Geometry: final body of the model. Coordinates: model frame, mm. Face numbers are marked on the shaded views. Round coordinates to 2 decimals unless told otherwise and drop trailing zeros. Loops run counter-clockwise (first coordinate to the right, second up) from the corner with the lowest first, then second, coordinate; pieces in that order, holes last. Notation, with made-up numbers: (12, 89.25) - (53, 89.25) arc R15 ccw to (53, 97.25) - close; hole circle Ø9 at (80, 9.5). An arc over 180 degrees is marked (long way). Answer as CSV lines item,"result".
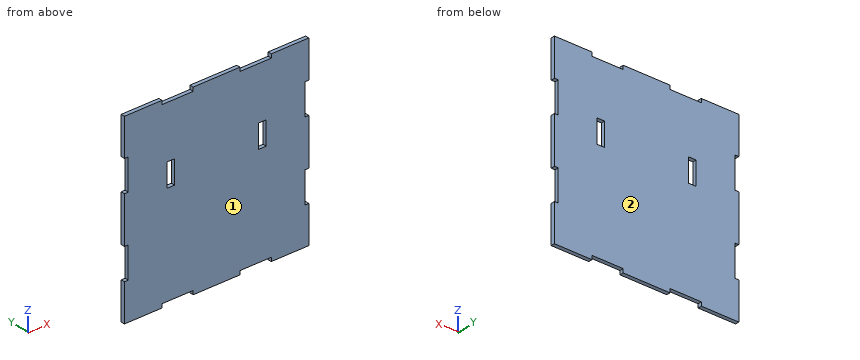
from build123d import *

# Parameters (mm, degrees)
CROQUIS1_W              = 4.84
CROQUIS1_H              = 15
SALIENTE_EXTRUIR1_DEPTH = 2.44


with BuildPart() as part:
    # Croquis1 → Saliente-Extruir1 (new body)
    with BuildSketch(Plane(origin=(0, 0, 0), x_dir=(1, 0, 0), z_dir=(0, 1, 0))):
        Polygon((-59, -59), (-35, -59), (-35, -56.56), (-15, -56.56), (-15, -59), (15, -59), (15, -56.56), (35, -56.56), (35, -59), (59, -59), (59, -35), (56.56, -35), (56.56, -15), (59, -15), (59, 15), (56.56, 15), (56.56, 35), (59, 35), (59, 59), (35, 59), (35, 56.56), (15, 56.56), (15, 59), (-15, 59), (-15, 56.56), (-35, 56.56), (-35, 59), (-59, 59), (-59, 35), (-56.56, 35), (-56.56, 15), (-59, 15), (-59, -15), (-56.56, -15), (-56.56, -35), (-59, -35), align=None)
        with Locations((-29.32, -15.28)):
            Rectangle(CROQUIS1_W, CROQUIS1_H, mode=Mode.SUBTRACT)
        with Locations((29.32, -15.28)):
            Rectangle(CROQUIS1_W, CROQUIS1_H, mode=Mode.SUBTRACT)
    extrude(amount=SALIENTE_EXTRUIR1_DEPTH)


solid = part.part
(1) Section B-B (x = 22). Output: boundary loops of the cut face in (y, z).
Findings below:
outline,"(0, -56.56) - (2.44, -56.56) - (2.44, 56.56) - (0, 56.56) - close"
(2) Pin query (flat end, axial travel): P1, Ø1.2, axis at y = 1.5, z = 17.5, coming from the +X side; P2, Ø1.2, axis at x = -24, y = 1.5, coming from the +Z side; P3, Ø0.7, axis at y = 1, z = 20, coming from the -X side. Return the tip coordinate at first contact, or that it passes through.
Findings below:
P1,"x = 56.56"
P2,"z = 56.56"
P3,"x = -56.56"
(3) Draft query along Y for the marked faces 1 and 2. Return one class per face: pulls with the +Y half, pulls with the -Y half, needs draft (parallel to the pull), parting line crosses it, or undercut.
Findings below:
face 1,"pulls with the -Y half"
face 2,"pulls with the +Y half"
(4) Material intervals for line 1 along X through (y, z) = (1.8, 18); line 2 along Z through (x, y) = (-30, 2.3); line 3 along Z through (x, y) = (22, 2.35), sorted ascending.
Findings below:
line 1,"-56.56 to -31.74, -26.9 to 26.9, 31.74 to 56.56"
line 2,"-56.56 to 7.78, 22.78 to 56.56"
line 3,"-56.56 to 56.56"
(5) Section A-A (y = 1.1). Give the number of separate pieces and of enclosed holes in the cut face, and give its area (3 significant figures).
Findings below:
separate pieces,"1"
enclosed holes,"2"
area,"13,400 mm2"
